Geometry: final body of the model. Coordinates: model frame, mm. Face numbers are marked on the shaded views. A direction names the side the tool comes from. Give positions to 0.01 mm unless a question says otherwise; leave off trailing zeros. One line per item, written item: value. Start each with the question number.
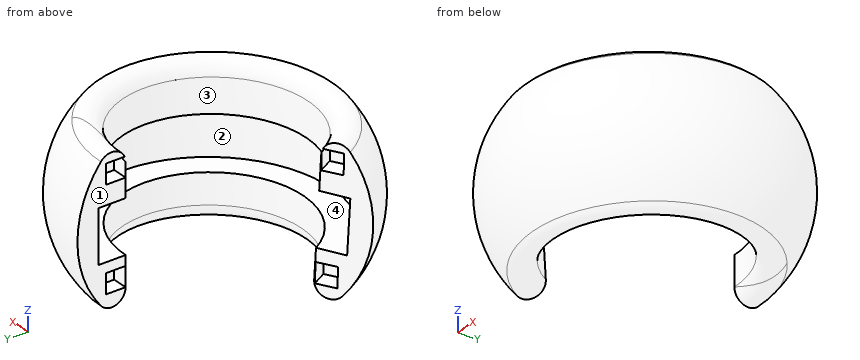
from build123d import *

# Parameters (mm, degrees)
F2_ANGLE    = 240
F3_W        = 7.112
F3_H        = 7.112
F4_DEPTH    = 5.55625
F5_W        = 7.112
F5_H        = 7.112
F6_DEPTH    = 5.55625
F7_T4_ANGLE = 349.948380696
F7_T9_ANGLE = 349.948380696
F8_T4_ANGLE = 343.9133898586
F8_T9_ANGLE = 343.9133898586
F11_DEPTH   = 6.35
F13_DEPTH   = 6.35


# Not quite as in the source:
# - a fillet or chamfer that OpenCascade refuses, or shapes differently, is made with other operations: its cross-section is extruded or revolved along the edge and cut away or added


with BuildPart() as f2:
    # F0 (on Right) → F2 (revolve)
    with BuildSketch(Plane.YZ):
        with BuildLine():
            Line((0, -25.9387402122), (0, -47.9325240122))
            ThreePointArc((0, -47.9325240122), (17.5731218804, -15.7507240122), (0, 16.4310759878))
            Line((0, 16.4310759878), (0, -6.8887402122))
            Line((0, -6.8887402122), (9.8796226174, -6.8887402122))
            Line((9.8796226174, -6.8887402122), (9.8796226174, -25.9387402122))
            Line((9.8796226174, -25.9387402122), (0, -25.9387402122))
        make_face()
    revolve(axis=Axis((0, -32.9686308407, -2.2695437855), (0, 0.0285596631, -0.9995920896)), revolution_arc=F2_ANGLE)

    # F3 (on Right) → F4 (cut)
    with BuildSketch(Plane.YZ):
        with Locations((3.556, 3.556)):
            Rectangle(F3_W, F3_H)
    extrude(amount=F4_DEPTH, mode=Mode.SUBTRACT)

    # F5 (on Right) → F6 (cut)
    with BuildSketch(Plane.YZ):
        with Locations((3.556, -33.1353539076)):
            Rectangle(F5_W, F5_H)
    extrude(amount=F6_DEPTH, mode=Mode.SUBTRACT)

    # F7: fillet of radius 5.08 on 1 edges, made by hand


with BuildPart() as f7_tool2:
    # F7_s3 → F7_t4 (revolve)
    with BuildSketch(Plane(origin=(-15.519406183, -22.1337407382, -0.6323901361), x_dir=(0.8187835052, -0.5741024052, 0), z_dir=(-0.5739453762, -0.8185595508, -0.0233873249))):
        with BuildLine():
            ThreePointArc((-13.6205038164, -36.4192771202), (-16.9439528127, -41.2478681872), (-22.6057068813, -39.7295975294))
            ThreePointArc((-22.6057068813, -39.7295975294), (-18.3618922347, -44.077312283), (-13.4832691044, -47.6983097543))
            Line((-13.4832691044, -47.6983097543), (-13.6205038164, -36.4192771202))
        make_face()
    revolve(axis=Axis((0, -31.638152468, -48.8364677143), (0, 0.0285596631, -0.9995920896)), revolution_arc=F7_T4_ANGLE)

    split(bisect_by=Plane.XZ, keep=Keep.TOP)


with BuildPart() as f2_1:
    add(f2.part)

    # F7_t1: cut F7_tool2
    add(f7_tool2.part, mode=Mode.SUBTRACT)


with BuildPart() as f7_tool7:
    # F7_s8 → F7_t9 (revolve)
    with BuildSketch(Plane(origin=(-15.519406183, -22.1337407382, -0.6323901361), x_dir=(0.8187835052, -0.5741024052, 0), z_dir=(-0.5739453762, -0.8185595508, -0.0233873249))):
        with BuildLine():
            ThreePointArc((-13.6205038164, -36.4192771202), (-16.9439528127, -41.2478681872), (-22.6057068813, -39.7295975294))
            ThreePointArc((-22.6057068813, -39.7295975294), (-18.3618922347, -44.077312283), (-13.4832691044, -47.6983097543))
            Line((-13.4832691044, -47.6983097543), (-13.6205038164, -36.4192771202))
        make_face()
    revolve(axis=Axis((0, -31.638152468, -48.8364677143), (0, 0.0285596631, -0.9995920896)), revolution_arc=F7_T9_ANGLE)

    split(bisect_by=Plane.XZ, keep=Keep.BOTTOM)


with BuildPart() as f2_2:
    add(f2_1.part)

    # F7_t6: cut F7_tool7
    add(f7_tool7.part, mode=Mode.SUBTRACT)

    # F8: fillet of radius 5.08 on 1 edges, made by hand


with BuildPart() as f8_tool2:
    # F8_s3 → F8_t4 (revolve)
    with BuildSketch(Plane(origin=(-16.0256017919, -20.4715562588, -0.5848993354), x_dir=(0.7874231543, -0.6164128292, 0), z_dir=(-0.6162568906, -0.7872239539, -0.0224920256))):
        with BuildLine():
            ThreePointArc((-12.7256800931, 5.3739698626), (-16.1598904571, 10.124422904), (-21.7850242933, 8.4756432802))
            ThreePointArc((-21.7850242933, 8.4756432802), (-17.6428750877, 12.9203239541), (-12.8492834764, 16.6531601142))
            Line((-12.8492834764, 16.6531601142), (-12.7256800931, 5.3739698626))
        make_face()
    revolve(axis=Axis((0, -33.4756053748, 15.4746338351), (0, 0.0285596631, -0.9995920896)), revolution_arc=F8_T4_ANGLE)

    split(bisect_by=Plane.XZ, keep=Keep.TOP)


with BuildPart() as f2_3:
    add(f2_2.part)

    # F8_t1: cut F8_tool2
    add(f8_tool2.part, mode=Mode.SUBTRACT)


with BuildPart() as f8_tool7:
    # F8_s8 → F8_t9 (revolve)
    with BuildSketch(Plane(origin=(-16.0256017919, -20.4715562588, -0.5848993354), x_dir=(0.7874231543, -0.6164128292, 0), z_dir=(-0.6162568906, -0.7872239539, -0.0224920256))):
        with BuildLine():
            ThreePointArc((-12.7256800931, 5.3739698626), (-16.1598904571, 10.124422904), (-21.7850242933, 8.4756432802))
            ThreePointArc((-21.7850242933, 8.4756432802), (-17.6428750877, 12.9203239541), (-12.8492834764, 16.6531601142))
            Line((-12.8492834764, 16.6531601142), (-12.7256800931, 5.3739698626))
        make_face()
    revolve(axis=Axis((0, -33.4756053748, 15.4746338351), (0, 0.0285596631, -0.9995920896)), revolution_arc=F8_T9_ANGLE)

    split(bisect_by=Plane.XZ, keep=Keep.BOTTOM)


with BuildPart() as f2_4:
    add(f2_3.part)

    # F8_t6: cut F8_tool7
    add(f8_tool7.part, mode=Mode.SUBTRACT)

    # F10 (on offset) → F11 (cut)
    with BuildSketch(Plane(origin=(14.2980794165, -24.7548980996, -0.7072800555), x_dir=(-0.8660254038, -0.4997960448, -0.0142798315), z_dir=(-0.5, 0.865672143, 0.0247333937))):
        Polygon((49.7467838827, 7.2109422366), (49.8148426414, 0), (56.9025047774, 0), (56.9025047774, 7.2109422366), align=None)
    extrude(amount=-F11_DEPTH, mode=Mode.SUBTRACT)

    # F12 (on offset) → F13 (cut)
    with BuildSketch(Plane(origin=(14.2980794165, -24.7548980996, -0.7072800555), x_dir=(-0.8660254038, -0.4997960448, -0.0142798315), z_dir=(-0.5, 0.865672143, 0.0247333937))):
        Polygon((55.8907425518, -30.6380988543), (48.7787425518, -30.6380988543), (48.716083169, -37.7500988543), (55.8907425518, -37.7500988543), align=None)
    extrude(amount=-F13_DEPTH, mode=Mode.SUBTRACT)


solid = f2_4.part
Item 1: Mould query, pull axis X, two halves, no side actions, for the marked faces 1 and 2. Classes: pulls with the +X half, pulls with the -X half, needs draft (parallel to the pull), parting line crosses it, or undercut.
Item 2: Pin query (flat end, axial travel): pin 1 (10 mm diameter, centred on x = -11, z = -15.5, fed in from +Y); pin 2 (2 mm diameter, centred on y = -49.5, z = 2, fed in from +X); pin 3 (8 mm diameter, centred on y = 2.5, z = -32.5, fed in from -X); pin 4 (10 mm diameter, centred on x = 39.5, y = 6, fed in from +Z). Return the tip coordinate at first contact, or that it passes through.
Item 3: Access query for the marked faces 3 and 4. Directions: +Z, -Z, +X, -X, +Y, -Y. A direction counts if a zero-diameter tool reaches every point of the face in a straight line with its end or side. Return the directions, or none.
Item 4: Ray query, line 1 along Z through (x, y) = (20.5, -5); line 2 along X through (y, z) = (-59.5, -18.5); line 3 along X through (y, z) = (-52, -7). Return the intervals inside material, ascending. Write a range as [from, to].
Geometry check:
1. face 1: pulls with the -X half
1. face 2: undercut
2. pin 1: stops at y = -71.98
2. pin 2: stops at x = 42.96
2. pin 3: stops at x = 0
2. pin 4: passes through
3. face 3: +Z
3. face 4: none
4. line 1: z = [-40.83, -26.13], [-7.08, 8.71]
4. line 2: x = [-42.23, -32.74], [32.74, 42.23]
4. line 3: x = [-33.18, -26.7], [26.7, 45.01]
